from build123d import *

# Parameters (mm, degrees)
SKETCH1_W           = 50
SKETCH1_H           = 36
SKETCH1_R           = 1.25
SKETCH1_R_2         = 1.7
BOSS_EXTRUDE1_DEPTH = 3.175


with BuildPart() as part:
    # Sketch1 → Boss-Extrude1 (new body)
    with BuildSketch(Plane(origin=(0, 0, 0), x_dir=(1, 0, 0), z_dir=(0, 1, 0))):
        with Locations((25, 18)):
            Rectangle(SKETCH1_W, SKETCH1_H)
        with Locations((13, 6.5)):
            Circle(SKETCH1_R, mode=Mode.SUBTRACT)
        with Locations((5, 5)):
            Circle(SKETCH1_R_2, mode=Mode.SUBTRACT)
        with Locations((5, 31)):
            Circle(SKETCH1_R_2, mode=Mode.SUBTRACT)
        with Locations((45, 31)):
            Circle(SKETCH1_R_2, mode=Mode.SUBTRACT)
        with Locations((45, 5)):
            Circle(SKETCH1_R_2, mode=Mode.SUBTRACT)
        with Locations((23, 6.5)):
            Circle(SKETCH1_R, mode=Mode.SUBTRACT)
        with Locations((33, 6.5)):
            Circle(SKETCH1_R, mode=Mode.SUBTRACT)
        with Locations((23, 16.5)):
            Circle(SKETCH1_R, mode=Mode.SUBTRACT)
        with Locations((33, 16.5)):
            Circle(SKETCH1_R, mode=Mode.SUBTRACT)
        with Locations((23, 26.5)):
            Circle(SKETCH1_R, mode=Mode.SUBTRACT)
        with Locations((33, 26.5)):
            Circle(SKETCH1_R, mode=Mode.SUBTRACT)
        with Locations((13, 16.5)):
            Circle(SKETCH1_R, mode=Mode.SUBTRACT)
        with Locations((13, 26.5)):
            Circle(SKETCH1_R, mode=Mode.SUBTRACT)
    extrude(amount=BOSS_EXTRUDE1_DEPTH)


solid = part.part
Geometry: final body of the model. Coordinates: model frame, mm. Round coordinates to 2 decimals unless told otherwise and drop trailing zeros. Loops run counter-clockwise (first coordinate to the right, second up) from the corner with the lowest first, then second, coordinate; pieces in that order, holes last. Notation, with made-up numbers: (31, 5) - (50, 5) arc R17 cw to (50, 18) - close; hole circle Ø6 at (52.5, 59). An arc over 180 degrees is marked (long way). Write each question's results on one line, items separated by ' | '. Start each with the question number.
1) Cut plane D-D on y = 2.35. Count the separate pieces of the cut face and the enclosed holes in it, then the cut area to 3 significant figures.
2) Cut plane C-C on z = -31. Return loops of the section in (x, y) (3 decimals), then the cut area to 3 significant figures.
3) First-contact query: P1, Ø1.5, axis at x = 13, z = -6.5, coming from the -Y side; P2, Ø3, axis at x = 23, z = -26.5, coming from the -Y side. Flat tips, straight axial feed; report the tip coordinate or a pass-through.
4) Cut plane B-B on x = 5. Return loops of the section in (y, z) (3 decimals), then the cut area to 3 significant figures.
5) Line query: probe 1 along Z at (x, y) = (23, 1.4); probe 2 along X at (y, z) = (1.6, -26.5); probe 3 along X at (y, z) = (1.1, -5). Output: solid intervals per line, ascending. Write a range as [from, to].
6) Mould query, pull axis Z, two halves, no side actions, for faces 1 (the face through (5.8, 1.6, -3.5)), 2 (the face through (24.155, 1.565, -6.021)), 3 (the face through (25, 2, 0)), 4 (the face through (25, 2, -36)). Classes: released by +Z, released by -Z, zero draft, split by the parting line, or undercut.
7) Cut plane A-A on x = 33. Return loops of the section in (y, z) (3 decimals), then the cut area to 3 significant figures.
Verdict:
1) separate pieces: 1 | enclosed holes: 13 | area: 1,720 mm2
2) outline: (0, 0) - (3.3, 0) - (3.3, 3.175) - (0, 3.175) - close; (6.7, 0) - (43.3, 0) - (43.3, 3.175) - (6.7, 3.175) - close; (46.7, 0) - (50, 0) - (50, 3.175) - (46.7, 3.175) - close | area: 137 mm2
3) P1: passes through | P2: stops at y = 0
4) outline: (0, -36) - (3.175, -36) - (3.175, -32.7) - (0, -32.7) - close; (0, -29.3) - (3.175, -29.3) - (3.175, -6.7) - (0, -6.7) - close; (0, -3.3) - (3.175, -3.3) - (3.175, 0) - (0, 0) - close | area: 92.7 mm2
5) probe 1: z = [-36, -27.75], [-25.25, -17.75], [-15.25, -7.75], [-5.25, 0] | probe 2: x = [0, 11.75], [14.25, 21.75], [24.25, 31.75], [34.25, 50] | probe 3: x = [0, 3.3], [6.7, 43.3], [46.7, 50]
6) face 1: undercut | face 2: undercut | face 3: released by +Z | face 4: released by -Z
7) outline: (0, -36) - (3.175, -36) - (3.175, -27.75) - (0, -27.75) - close; (0, -25.25) - (3.175, -25.25) - (3.175, -17.75) - (0, -17.75) - close; (0, -15.25) - (3.175, -15.25) - (3.175, -7.75) - (0, -7.75) - close; (0, -5.25) - (3.175, -5.25) - (3.175, 0) - (0, 0) - close | area: 90.5 mm2
